Could you check a few things on this model? Use its own coordinates, in mm. A direction names the side the tool comes from. Give positions to 0.01 mm unless a question says otherwise; leave off trailing zeros. Loops run counter-clockwise (first coordinate to the right, second up) from the corner with the lowest first, then second, coordinate; pieces in that order, holes last. Notation, with made-up numbers: M -33.5,87 L -2.5,87 A10 ccw -2.5,103 Z; hole C 25.25,-11 d3. An arc over 180 degrees is marked long. Use a Markdown table: item, result. Add a question column.
1) Suppose I cut it at A-A on z = -27. List the corners of the cut face in (x, y) for me, and give its area (3 significant figures).
2) If I drill on line 1 along X through (y, z) = (12, -29.75); line 2 along X through (y, z) = (14, -25.5); line 3 along Z through (x, y) = (27, 62), over which ranges is the centre line in solid material (lowest first)? Write a range as [from, to].
3) Suppose I cut it at D-D on z = -20.75. List the corners of the cut face in (x, y) for me.
4) Which directions (+Z, -Z, +X, -X, +Y, -Y) give clear straight access to the entire face, cutting with the end or side of a thin tool? Please do faces 4 (the flat face through (24.203, 36, -24)), 5 (the flat face through (-17, 36, -17.698)), 6 (the flat face through (6, 36, -14.523)).
5) We'd pull the mould along X, two halves only. Please class faces 1 (the flat face through (36.903, 36, -16)), 2 (the flat face through (-23.849, 36, -16)), 3 (the cylindrical face through (6.8, 61.7, -17.7)): +X half, -X half, draft (parallel to the pull), parting line (faces both ways), or undercut.
6) Suppose I cut it at B-B on y = 39.5. List the corners of the cut face in (x, z) for me (3 decimals).
7) Will these pins go through, and if not, where does the flat tip stop? pin 1 Ø5 at (y, z) = (29.5, -28.5) entering from +X; pin 2 Ø6 at (y, z) = (64.5, -23.5) entering from -X; pin 3 Ø10 at (x, y) = (-19.5, 39.5) entering from -Z.
8) Suppose I cut it at C-C on x = 6. List the corners of the cut face in (y, z) for me.
```python
from build123d import *

# Parameters (mm, degrees)
BOSS_EXTRUDE3_DEPTH = 72.39
BOSS_EXTRUDE4_DEPTH = 51.39


with BuildPart() as part:
    # Sketch1 → Boss-Extrude3 (new body)
    with BuildSketch(Plane(origin=(0, 0, 0), x_dir=(1, 0, 0), z_dir=(0, 1, 0))):
        with BuildLine():
            Line((-11.1466884, 17.698170271), (-23.8485284, 17.698170271))
            Line((-23.8485284, 17.698170271), (-23.8485284, 14.523170271))
            Line((-23.8485284, 14.523170271), (36.9033116, 14.523170271))
            Line((36.9033116, 14.523170271), (36.9033116, 17.698170271))
            Line((36.9033116, 17.698170271), (24.2033116, 17.698170271))
            Line((24.2033116, 17.698170271), (24.2033116, 31.198170271))
            Line((24.2033116, 31.198170271), (20.025, 31.198170271))
            ThreePointArc((20.025, 31.198170271), (6.525, 17.69817027), (-6.975, 31.198170271))
            Line((-6.975, 31.198170271), (-11.1466884, 31.198170271))
            Line((-11.1466884, 31.198170271), (-11.1466884, 17.698170271))
        make_face()
    extrude(amount=BOSS_EXTRUDE3_DEPTH)

    # Sketch1<13> → Boss-Extrude4 (add)
    with BuildSketch(Plane(origin=(0, 0, 0), x_dir=(1, 0, 0), z_dir=(0, 1, 0))):
        with BuildLine():
            Line((-6.975, 31.198170271), (-6.675, 31.198170271))
            ThreePointArc((-6.675, 31.198170271), (6.525, 17.99817027), (19.725, 31.198170271))
            Line((19.725, 31.198170271), (20.025, 31.198170271))
            ThreePointArc((20.025, 31.198170271), (6.525, 17.69817027), (-6.975, 31.198170271))
        make_face()
    extrude(amount=BOSS_EXTRUDE4_DEPTH)


solid = part.part
```
Answer block:
| question | item | result |
|---|---|---|
| 1 | outline | M -11.15,0 L -5.99,0 L -5.99,51.39 L -6.31,51.39 L -6.31,72.39 L -11.15,72.39 Z; M 19.04,0 L 24.2,0 L 24.2,72.39 L 19.36,72.39 L 19.36,51.39 L 19.04,51.39 Z |
| 1 | area | 734 mm^2 |
| 2 | line 1 | x = [-11.15, -6.6], [19.65, 24.2] |
| 2 | line 2 | x = [-11.15, -5.38], [18.43, 24.2] |
| 2 | line 3 | z = [-17.7, -14.52] |
| 3 | outline | M -11.15,0 L -1.54,0 L -1.54,51.39 L -2.02,51.39 L -2.02,72.39 L -11.15,72.39 Z; M 14.59,0 L 24.2,0 L 24.2,72.39 L 15.07,72.39 L 15.07,51.39 L 14.59,51.39 Z |
| 4 | face 4 | -Z, +X, +Y, -Y |
| 4 | face 5 | -Z, -X, +Y, -Y |
| 4 | face 6 | +Z, +X, -X, +Y, -Y |
| 5 | face 1 | +X half |
| 5 | face 2 | -X half |
| 5 | face 3 | undercut |
| 6 | outline | M -23.849,-17.698 L -11.147,-17.698 L -11.147,-31.198 L -6.675,-31.198 A13.2 cw 19.725,-31.198 L 24.203,-31.198 L 24.203,-17.698 L 36.903,-17.698 L 36.903,-14.523 L -23.849,-14.523 Z |
| 7 | pin 1 | stops at x = 24.2 |
| 7 | pin 2 | stops at x = -11.15 |
| 7 | pin 3 | stops at z = -17.7 |
| 8 | outline | M 0,-18.01 L 51.39,-18.01 L 51.39,-17.71 L 72.39,-17.71 L 72.39,-14.52 L 0,-14.52 Z |
